The listing builds one solid part. Answer for the finished solid, in the listing's coordinates (mm). A direction names the side the tool comes from. Give positions to 0.01 mm unless a question says otherwise; leave off trailing zeros. Order: outer loops, then holes, each group sorted by start corner. A loop starts at its lowest first (then second) coordinate and runs counter-clockwise, first axis right, second up. Notation, with made-up numbers: (-3, 81) - (23, 81) arc R32 ccw to (23, 109) - close; hole circle Ø4 at (86.25, -29). An arc over 180 degrees is marked (long way). Answer as a JSON object with one key per item and string values. Group by question number.
Q1. A cutting plane is placed at D-D, the plane z = 32.5. Give the vertices of the cut face in (x, y), and give its area (3 significant figures).
Q2. A cutting plane is placed at A-A, the plane y = 0. Give the vertices of the cut face in (x, z), and give its area (3 significant figures).
Q3. The mould has two halves that part along Y. Classify faces 4 (the face through (19, -2, 0)), 5 (the face through (17, -3, 20)), 6 (the face through (0, -2, 21)): released by +Y, released by -Y, zero draft, split by the parting line, or undercut.
Q4. Consider line 1 (Y direction, x = 0, z = 26); line 2 (Y direction, x = 13, z = 16). Determine where each line is inside the solid, lowest interval first.
Q5. For faces 1 (the face through (19, -2, 40)), 2 (the face through (4.943, -2, 35)), 3 (the face through (2, -1, 10.762)), determine the directions among +Z, -Z, +X, -X, +Y, -Y from which every point of the face is accessible in a straight line to the end or side of a thin tool.
Q6. A cutting plane is placed at C-C, the plane x = 31.5. Give the vertices of the cut face in (y, z).
Q7. Given pin 1 (3 mm diameter, centred on x = 3, y = 0.5, fed in from +Z); pin 2 (9 mm diameter, centred on x = 22.5, z = 12.5, fed in from +Y); pin 3 (0.6 mm diameter, centred on y = -2, z = 7.5, fed in from -X); pin 4 (1 mm diameter, centred on x = 16.5, y = 0, fed in from +Z), each flat-ended and moving along its own axis, determine where each tip first touches the part or whether it passes through.
Q8. A cutting plane is placed at B-B, the plane z = 28. Give the vertices of the cut face in (x, y), and give its area (3 significant figures).
from build123d import *

# Parameters (mm, degrees)
SKETCH_1_R          = 2
EXTRUDE_1_DEPTH     = 40
SKETCH_2_W          = 10.776638496
SKETCH_2_H          = 12.262488547
SKETCH_2_H_2        = 11.437792605
CUT_EXTRUDE_2_DEPTH = 20


with BuildPart() as part:
    # Эскиз1 → Вытянуть1 (new body)
    with BuildSketch(Plane.XY):
        with BuildLine():
            Line((2.828427125, -1), (32.828427125, -1))
            Line((32.828427125, -1), (32.828427125, -3))
            Line((32.828427125, -3), (0, -3))
            ThreePointArc((0, -3), (-1.732050808, 2.449489743), (2.828427125, -1))
        make_face()
        Circle(SKETCH_1_R, mode=Mode.SUBTRACT)
    extrude(amount=EXTRUDE_1_DEPTH)

    # Эскиз2 → Вытянуть2 (cut, symmetric)
    with BuildSketch(Plane(origin=(0, 0, 0), x_dir=(1, 0, 0), z_dir=(0, 1, 0))):
        with Locations((-0.445273779, -4.631244274)):
            Rectangle(SKETCH_2_W, SKETCH_2_H)
        with Locations((-0.445273779, -36.556842192)):
            Rectangle(SKETCH_2_W, SKETCH_2_H_2)
    extrude(amount=CUT_EXTRUDE_2_DEPTH, both=True, mode=Mode.SUBTRACT)


solid = part.part
Reply:
{
 "1": {"outline": "(4.94, -3) - (32.83, -3) - (32.83, -1) - (4.94, -1) - close", "area": "55.8 mm^2"},
 "2": {"outline": "(-3, 10.76) - (-2, 10.76) - (-2, 30.84) - (-3, 30.84) - close; (2, 10.76) - (3, 10.76) - (3, 30.84) - (2, 30.84) - close", "area": "40.2 mm^2"},
 "3": {"face 4": "zero draft", "face 5": "released by -Y", "face 6": "undercut"},
 "4": {"line 1": "y = -3 to -2, 2 to 3", "line 2": "y = -3 to -1"},
 "5": {"face 1": "+Z, +X, -X, +Y, -Y", "face 2": "+Z, -X, +Y, -Y", "face 3": "-Z, -X, +Y, -Y"},
 "6": {"outline": "(-3, 0) - (-1, 0) - (-1, 40) - (-3, 40) - close"},
 "7": {"pin 1": "stops at z = 30.84", "pin 2": "stops at y = -1", "pin 3": "stops at x = 4.94", "pin 4": "passes through"},
 "8": {"outline": "(0, -3) - (32.83, -3) - (32.83, -1) - (2.83, -1) arc R3 ccw (long way) to start; hole circle Ø4 at (0, 0)", "area": "77.2 mm^2"}
}
